Study the drawing (mm; zero at the part's minimum x, y, z) and answer. A direction names the side the tool comes from. Coordinates: 2 decimals unless noted, no trailing zeros. Loops run counter-clockwise (first coordinate to the right, second up) from the corner with the lowest first, then second, coordinate; pieces in that order, holes last. Notation, with made-up numbers: (46.25, 29) - (67.25, 29) arc R10 cw to (67.25, 48) - close; hole circle Ø3 at (-1, -17.5). An arc over 180 degrees is marked (long way). Put each result on its own line as item: value.
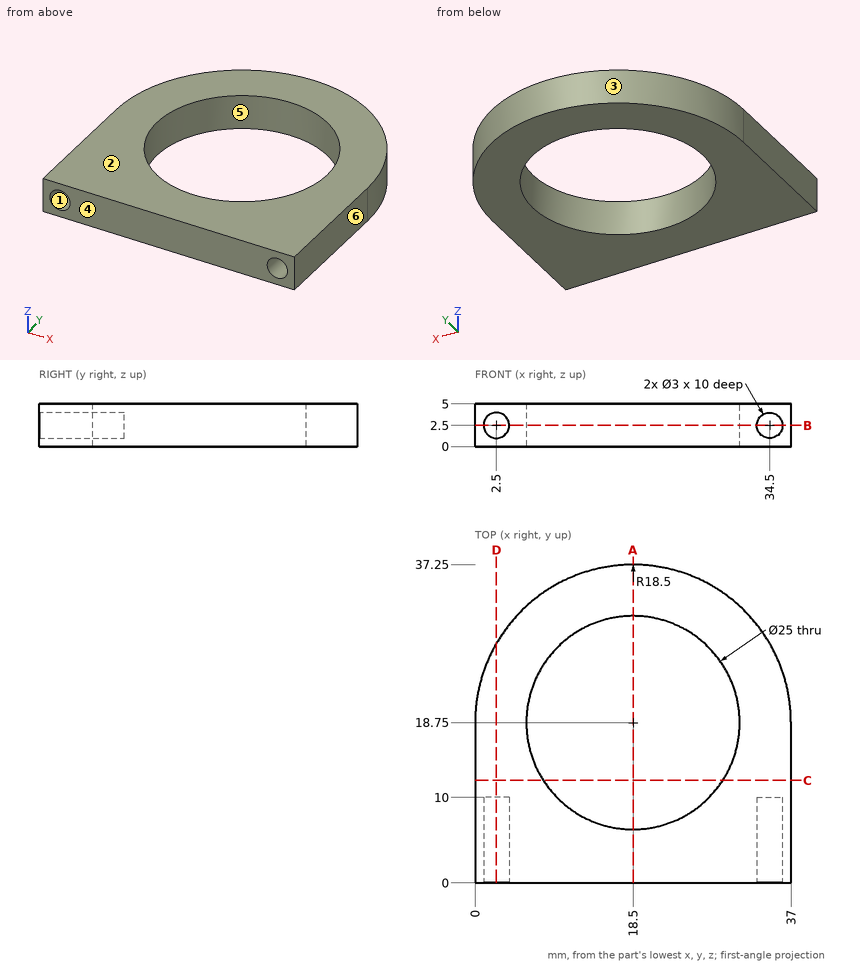
1) For a pull along X with two mould halves and no side action, classify the marked faces 3, 4, 5 and 6 as pulls with the +X half, pulls with the -X half, needs draft (parallel to the pull), parting line crosses it, or undercut.
Found:
face 3: parting line crosses it
face 4: needs draft
face 5: undercut
face 6: pulls with the +X half
2) The part is cut by section A-A (x = 18.5). Give the vertices of the cut face in (y, z).
Found:
outline: (0, 0) - (6.25, 0) - (6.25, 5) - (0, 5) - close; (31.25, 0) - (37.25, 0) - (37.25, 5) - (31.25, 5) - close
3) Each of these flat-tipped pins is pushed along its axis until it touches: pin 1 (2 mm diameter, centred on x = 31, z = 2.5, fed in from +Y); pin 2 (1.8 mm diameter, centred on x = 34.5, z = 2.5, fed in from -Y). Where does it stop, or does it pass through?
Found:
pin 1: stops at y = 33.24
pin 2: stops at y = 10
4) Straight lines are drawn through the part: L1, parallel to X at y = 2.5, z = 2.5; L2, parallel to Z at x = 34.5, y = 5.25; L3, parallel to X at y = 18.5, z = 3.6. For each, find the intervals that lie inside material, in ascending order. Write a range as [from, to].
Found:
L1: x = [0, 1], [4, 33], [36, 37]
L2: z = [0, 1], [4, 5]
L3: x = [0, 6], [31, 37]
5) The part is cut by section C-C (y = 12). Give the vertices of the cut face in (x, z).
Found:
outline: (0, 0) - (7.98, 0) - (7.98, 5) - (0, 5) - close; (29.02, 0) - (37, 0) - (37, 5) - (29.02, 5) - close
6) The part is cut by section D-D (x = 2.5). Give the vertices of the cut face in (y, z).
Found:
outline: (0, 0) - (28.04, 0) - (28.04, 5) - (0, 5) - (0, 4) - (10, 4) - (10, 1) - (0, 1) - close
7) For the marked faces 1 and 2, determine the directions among +Z, -Z, +X, -X, +Y, -Y from which every point of the face is accessible in a straight line to the end or side of a thin tool.
Found:
face 1: -Y
face 2: +Z, +X, -X, +Y, -Y
8) The part is cut by section B-B (z = 2.5). Give the vertices of the cut face in (x, y).
Found:
outline: (0, 0) - (1, 0) - (1, 10) - (4, 10) - (4, 0) - (33, 0) - (33, 10) - (36, 10) - (36, 0) - (37, 0) - (37, 18.75) arc R18.5 ccw to (0, 18.75) - close; hole circle Ø25 at (18.5, 18.75)
